Could you check a few things on this model? Use its own coordinates, in mm. A direction names the side the tool comes from. Give positions to 0.01 mm unless a question says otherwise; leave off trailing zeros. Write each loop counter-clockwise with the first axis right and the second up, starting at its lowest first coordinate (ties: lowest second). Pieces come first, ordered by that corner, then holes. Notation, with made-up numbers: (-17.5, 63) - (-2.5, 63) arc R18 cw to (-2.5, 84) - close; hole circle Ø11 at (55.5, 43). An arc over 180 degrees is marked (long way). Answer in a Markdown table with one row per item.
from build123d import *

# Parameters (mm, degrees)
F0_R     = 5
F0_R_2   = 10
F1_DEPTH = 25


with BuildPart() as f1:
    # F0 (on Top) → F1 (new body)
    with BuildSketch(Plane.XY):
        with BuildLine():
            Line((-30.551076, -35.12097), (19.448924, -35.12097))
            ThreePointArc((19.448924, -35.12097), (29.448924, -25.12097), (19.448924, -15.12097))
            Line((19.448924, -15.12097), (-20.551076, -15.12097))
            ThreePointArc((-20.551076, -15.12097), (-24.086609, -13.656504), (-25.551076, -10.12097))
            ThreePointArc((-25.551076, -10.12097), (-24.495347, -5.648834), (-21.551076, -2.12097))
            ThreePointArc((-21.551076, -2.12097), (-30.551076, 24.87903), (-39.551076, -2.12097))
            ThreePointArc((-39.551076, -2.12097), (-36.606804, -5.648834), (-35.551076, -10.12097))
            Line((-35.551076, -10.12097), (-35.551076, -11.892213))
            ThreePointArc((-35.551076, -11.892213), (-36.196932, -15.427747), (-38.051076, -18.506592))
            ThreePointArc((-38.051076, -18.506592), (-39.665454, -29.235348), (-30.551076, -35.12097))
        make_face()
        with Locations((-30.551076, -25.12097)):
            Circle(F0_R, mode=Mode.SUBTRACT)
        with Locations((19.448924, -25.12097)):
            Circle(F0_R, mode=Mode.SUBTRACT)
        with Locations((-30.551076, 9.87903)):
            Circle(F0_R_2, mode=Mode.SUBTRACT)
    extrude(amount=F1_DEPTH)


solid = f1.part
1) On a 3-axis mill with a long thin cutter (end or side, diameter ignored), from which of +Z, -Z, +X, -X, +Y, -Y can I reach the whole of each face in a straight line? I mean faces 4 (the face through (-35.551, -11, 12)), 5 (the face through (18.798, -20.164, 12.325)), 6 (the face through (-24.048, -13.695, 12.325)). Say none if no direction works.
Check values:
| item | result |
|---|---|
| face 4 | +Z, -Z, -X |
| face 5 | +Z, -Z |
| face 6 | +Z, -Z, +X |
2) Imagine slicing it at C-C (y = 7). List the corners of the cut face in (x, z) for me.
Check values:
| item | result |
|---|---|
| outline | (-45.27, 0) - (-40.13, 0) - (-40.13, 25) - (-45.27, 25) - close; (-20.97, 0) - (-15.83, 0) - (-15.83, 25) - (-20.97, 25) - close |
3) Imagine slicing it at D-D (z = 22). List the corners of the cut face in (x, y) for me.
Check values:
| item | result |
|---|---|
| outline | (-39.55, -2.12) arc R10 cw to (-35.55, -10.12) - (-35.55, -11.89) arc R10 cw to (-38.05, -18.51) arc R10 ccw to (-30.55, -35.12) - (19.45, -35.12) arc R10 ccw to (19.45, -15.12) - (-20.55, -15.12) arc R5 cw to (-25.55, -10.12) arc R10 cw to (-21.55, -2.12) arc R15 ccw (long way) to start; hole circle Ø20 at (-30.55, 9.88); hole circle Ø10 at (-30.55, -25.12); hole circle Ø10 at (19.45, -25.12) |
4) Imagine slicing it at A-A (x = -17). List the corners of the cut face in (y, z) for me.
Check values:
| item | result |
|---|---|
| outline | (-35.12, 0) - (-15.12, 0) - (-15.12, 25) - (-35.12, 25) - close; (3.45, 0) - (16.31, 0) - (16.31, 25) - (3.45, 25) - close |
5) If I drill on line 1 (X direction, y = -25.5, z = 22.75); line 2 (Y direction, x = -28, z = 6.75); line 3 (Y direction, x = -27, z = 10), over which ranges is the centre line in solid material (lowest first)?
Check values:
| item | result |
|---|---|
| line 1 | x = -40.54 to -35.54, -25.57 to 14.46, 24.43 to 29.44 |
| line 2 | y = -35.12 to -29.42, -20.82 to 0.21, 19.55 to 24.66 |
| line 3 | y = -35.12 to -28.64, -21.6 to 0.53, 19.23 to 24.45 |
6) Imagine slicing it at B-B (y = -28.5). List the corners of the cut face in (x, z) for me.
Check values:
| item | result |
|---|---|
| outline | (-39.96, 0) - (-34.24, 0) - (-34.24, 25) - (-39.96, 25) - close; (-26.87, 0) - (15.76, 0) - (15.76, 25) - (-26.87, 25) - close; (23.13, 0) - (28.86, 0) - (28.86, 25) - (23.13, 25) - close |
7) We'd pull the mould along X, two halves only. Please class faces 1 (the face through (-21.01, 12.88, 12.32)), 2 (the face through (-36.636, -5.591, 12.325)), 3 (the face through (-9, -18, 25)): +X half, -X half, draft (parallel to the pull), parting line (faces both ways), or undercut.
Check values:
| item | result |
|---|---|
| face 1 | undercut |
| face 2 | -X half |
| face 3 | draft |
8) Will these pins go through, and if not, where does the flat tip stop? P1, Ø1, axis at y = -4, z = 6, coming from the +X side; P2, Ø8, axis at x = -37, z = 10.5, coming from the +Y side; P3, Ø8, axis at x = 11, z = 14, coming from the +Y side.
Check values:
| item | result |
|---|---|
| P1 | stops at x = -23.05 |
| P2 | stops at y = 24.68 |
| P3 | stops at y = -15.12 |
